Autodesk Inventor part; units mm, degrees
ref_plane "YZ Plane" through (0, 0, 0) normal (1, 0, 0) x (0, 1, 0)
ref_plane "XZ Plane" through (0, 0, 0) normal (0, 1, 0) x (-1, 0, 0)
ref_plane "XY Plane" through (0, 0, 0) normal (0, 0, 1) x (1, 0, 0)
sketch "草图1" plane through (0, 0, 0) normal (0, 1, 0) x (-1, 0, 0)
  line L0 (-5, 0) -> (-170, 0)
  line L1 (-175, 5) -> (-175, 155)
  line L2 (-170, 160) -> (-5, 160)
  line L3 (0, 155) -> (0, 5)
  line L4 (22.306, 80) -> (-199.7113, 80)
  line L5 (-87.5, 206.246) -> (-87.5, -79.95)
  circle A0 centre (-10, 150) radius 4
  circle A1 centre (-10, 10) radius 4
  circle A2 centre (-165, 150) radius 4
  circle A3 centre (-165, 10) radius 4
  arc A4 (0, 155) -> (-5, 160) centre (-5, 155) ccw
  arc A5 (-5, 0) -> (0, 5) centre (-5, 5) ccw
  arc A6 (-175, 5) -> (-170, 0) centre (-170, 5) ccw
  arc A7 (-170, 160) -> (-175, 155) centre (-170, 155) ccw
  point P0 (0, 0)
  point P1 (-175, 0)
  point P2 (0, 160)
  point P3 (-87.5, 160)
  point P4 (0, 80)
  point P5 (-87.5, 80)
  point P6 (-87.5, 0)
  point P7 (-87.5, 80)
  dimension "d0" = 160
  dimension "d1" = 175
  dimension "d2" = 8
  dimension "d6" = 140
  dimension "d9" = 155
  dimension "d12" = 5
extrude "拉伸1" add sketch "草图1" along normal blind 8
sketch "草图2" plane through (0, 0, 0) normal (0, -1, 0) x (1, 0, 0)
  line L0 (150, 140) -> (25, 140)
  line L1 (20, 135) -> (20, 25)
  line L2 (25, 20) -> (150, 20)
  line L3 (155, 25) -> (155, 135)
  arc A0 (155, 135) -> (150, 140) centre (150, 135) ccw
  arc A1 (150, 20) -> (155, 25) centre (150, 25) ccw
  arc A2 (20, 25) -> (25, 20) centre (25, 25) ccw
  arc A3 (25, 140) -> (20, 135) centre (25, 135) ccw
  line L4 (87.5, 206.246) -> (87.5, -79.95)
  line L5 (-22.306, 80) -> (199.7113, 80)
  point P0 (0, 0)
  point P1 (87.5, 140)
  point P2 (155, 80)
  dimension "d15" = 5
  dimension "d16" = 120
  dimension "d17" = 135
extrude "拉伸2" cut sketch "草图2" against normal blind 1.5
fillet "圆角1" radius 2 8 edges at (153.5355, 1.5, 138.5355) (155, 1.5, 80) (153.5355, 1.5, 21.4645) (87.5, 1.5, 20) (21.4645, 1.5, 21.4645) (20, 1.5, 80) (21.4645, 1.5, 138.5355) (87.5, 1.5, 140)
sketch "草图3" plane through (0, 1.5, 0) normal (0, -1, 0) x (1, 0, 0)
  line L0 (71.5, 96) -> (103.5, 96)
  line L1 (103.5, 96) -> (103.5, 64)
  line L2 (103.5, 64) -> (71.5, 64)
  line L3 (71.5, 64) -> (71.5, 96)
  line L4 (-22.306, 80) -> (199.7113, 80)
  line L5 (87.5, 206.246) -> (87.5, -79.95)
  point P0 (0, 0)
  point P1 (71.5, 80)
  point P2 (87.5, 96)
  dimension "d28" = 32
extrude "拉伸3" add sketch "草图3" along normal blind 8.5
fillet "圆角2" radius 2 12 edges at (87.5, -7, 96) (103.5, -7, 80) (87.5, -7, 64) (71.5, -7, 80) (87.5, 1.5, 96) (71.5, 1.5, 80) (103.5, 1.5, 80) (87.5, 1.5, 64) (71.5, -2.75, 96) (71.5, -2.75, 64) (103.5, -2.75, 64) (103.5, -2.75, 96)
sketch "草图4" plane through (0, -7, 0) normal (0, -1, 0) x (1, 0, 0)
  line L0 (-22.306, 80) -> (199.7113, 80)
  line L1 (87.5, 206.246) -> (87.5, -79.95)
  point P0 (0, 0)
  point P1 (87.5, 80)
hole "孔2" at (87.5, -7, 80) direction (0, 1, 0) diameter 20.752 end through all
equation "\"d2\" = d4"
equation "\"d6\" = A2"
equation "\"d9\" = B2"
equation "\"d12\" = R"
equation "\"d13\" = h_"
equation "\"d15\" = R"
equation "\"d16\" = A_"
equation "\"d17\" = B"
properties part number "盖板" material "聚碳酸酯，透明"
Can you work these out from the model? Positions are in its coordinate system, mm. A direction names the side the tool comes from. Give positions to 0.01 mm unless a question says otherwise; leave off trailing zeros. Order: outer loops, then holes, each group sorted by start corner. A loop starts at its lowest first (then second) coordinate and runs counter-clockwise, first axis right, second up. Notation, with made-up numbers: (-5, -16.5) - (26, -16.5) arc R16 cw to (26, 4.5) - close; hole circle Ø4 at (-37.75, 61). An arc over 180 degrees is marked (long way). Use a Markdown table: item, result. Add a question column.
Q1. If we section it at A-A on x = 87.5: Write out the boundary of the cut face in (y, z).
Q2. If we section it at D-D on x = 10: Write out the boundary of the cut face in (y, z).
Q3. I'm going to push flat-ended pins straight in: pin 1 (2 mm diameter, centred on x = 81, y = -2.5, fed in from +Z); pin 2 (13 mm diameter, centred on x = 10, z = 150, fed in from -Y); pin 3 (12.5 mm diameter, centred on x = 87.5, z = 80, fed in from -Y); pin 4 (4 mm diameter, centred on y = 3, z = 91, fed in from -X). Where does each tip first touch, or does it pass through?
Q4. If we section it at C-C on z = 150: Write out the boundary of the cut face in (x, y).
Q5. If we section it at B-B on z = 80: Write out the boundary of the cut face in (x, y), plus the area to 3 significant figures.
Q6. On a 3-axis mill with a long thin cutter (end or side, diameter ignored), from which of +Z, -Z, +X, -X, +Y, -Y can I reach the whole of each face in a straight line? I mean faces 1 (the flat face through (88, -3, 64)), 2 (the flat face through (103.5, -3, 80)), 3 (the flat face through (87, 1.5, 107)). Say none if no direction works.
Q7. If we mould it in two halves opening along Z, with no side actions, what happens to faces 4 (the cylindrical face through (173, 4, 1)), 5 (the cylindrical face through (10.521, 3.944, 146.034)), 6 (the flat face through (87, -3, 96)), 7 (the flat face through (71.5, -3, 80))? For each: released by +Z, released by -Z, zero draft, split by the parting line, or undercut.
Q8. Please list where these lines run through material, in increasing order: line 1 along Z through (x, y) = (165, 4.75); line 2 along Z through (x, y) = (12.5, 4.5); line 3 along Y through (x, z) = (156, 116).
Answers follow:
| question | item | result |
|---|---|---|
| 1 | outline | (-7, 66) arc R2 ccw to (-5, 64) - (-0.5, 64) arc R2 cw to (1.5, 62) - (1.5, 21.94) arc R2 cw to (0, 20) - (0, 0) - (8, 0) - (8, 69.62) - (-7, 69.62) - close; (-7, 90.38) - (8, 90.38) - (8, 160) - (0, 160) - (0, 140) arc R2 cw to (1.5, 138.06) - (1.5, 98) arc R2 cw to (-0.5, 96) - (-5, 96) arc R2 ccw to (-7, 94) - close |
| 2 | outline | (0, 0) - (8, 0) - (8, 6) - (0, 6) - close; (0, 14) - (8, 14) - (8, 146) - (0, 146) - close; (0, 154) - (8, 154) - (8, 160) - (0, 160) - close |
| 3 | pin 1 | stops at z = 96 |
| 3 | pin 2 | stops at y = 0 |
| 3 | pin 3 | passes through |
| 3 | pin 4 | stops at x = 0 |
| 4 | outline | (0, 0) - (6, 0) - (6, 8) - (0, 8) - close; (14, 0) - (161, 0) - (161, 8) - (14, 8) - close; (169, 0) - (175, 0) - (175, 8) - (169, 8) - close |
| 5 | outline | (0, 0) - (20, 0) arc R2 cw to (21.94, 1.5) - (69.5, 1.5) arc R2 cw to (71.5, -0.5) - (71.5, -5) arc R2 ccw to (73.5, -7) - (77.12, -7) - (77.12, 8) - (0, 8) - close; (97.88, -7) - (101.5, -7) arc R2 ccw to (103.5, -5) - (103.5, -0.5) arc R2 cw to (105.5, 1.5) - (153.06, 1.5) arc R2 cw to (155, 0) - (175, 0) - (175, 8) - (97.88, 8) - close |
| 5 | area | 1,160 mm^2 |
| 6 | face 1 | -Z, +X, -X, -Y |
| 6 | face 2 | +Z, -Z, +X, -Y |
| 6 | face 3 | -Y |
| 7 | face 4 | released by -Z |
| 7 | face 5 | undercut |
| 7 | face 6 | released by +Z |
| 7 | face 7 | zero draft |
| 8 | line 1 | z = 0 to 6, 14 to 146, 154 to 160 |
| 8 | line 2 | z = 0 to 6.88, 13.12 to 146.88, 153.12 to 160 |
| 8 | line 3 | y = 0 to 8 |
